The listing builds one solid part. Answer for the finished solid, in the listing's coordinates (mm). A direction names the side the tool comes from. Round coordinates to 2 decimals unless told otherwise and drop trailing zeros. Loops run counter-clockwise (first coordinate to the right, second up) from the corner with the lowest first, then second, coordinate; pieces in that order, holes last. Notation, with made-up numbers: (-4, 41) -> (2, 41) arc R27 cw to (2, 57) -> close; hole circle Ø2 at (-27.5, 69). An arc over 180 degrees is marked (long way). One line per question, with ' | ' between items.
from build123d import *

# Parameters (mm, degrees)
PAD_DEPTH       = 40
SKETCH002_R     = 6.5
PAD001_DEPTH    = 3.25
SKETCH003_R     = 3.5
POCKET_DEPTH    = 8.251
SKETCH004_R     = 3
POCKET001_DEPTH = 5
CHAMFER_SIZE    = 2
FILLET_R        = 2
FILLET001_R     = 2
CHAMFER001_SIZE = 1


with BuildPart() as part:
    # Sketch → Pad (new body)
    with BuildSketch(Plane.XY):
        Polygon((0, 50), (0, 0), (-50, 0), (-50, 5), (-5, 5), (-5, 50), align=None)
    extrude(amount=PAD_DEPTH)

    # Sketch002 (on Face4 of Pad) → Pad001 (join)
    with BuildSketch(Plane(origin=(0, 5, 0), x_dir=(-1, 0, 0), z_dir=(0, 1, 0))):
        with Locations((25, 20)):
            Circle(SKETCH002_R)
    extrude(amount=PAD001_DEPTH)

    # Sketch003 (on Face10 of Pad001) → Pocket (cut, through all)
    with BuildSketch(Plane(origin=(0, 8.25, 0), x_dir=(-1, 0, 0), z_dir=(0, 1, 0))):
        with Locations((25, 20)):
            Circle(SKETCH003_R)
    extrude(amount=-POCKET_DEPTH, mode=Mode.SUBTRACT)

    # Sketch004 (on Face6 of Pocket) → Pocket001 (cut)
    with BuildSketch(Plane(origin=(-5, 0, 0), x_dir=(0, -1, 0), z_dir=(-1, 0, 0))):
        with Locations((-35, 30)):
            Circle(SKETCH004_R)
        with Locations((-20, 10)):
            Circle(SKETCH004_R)
    extrude(amount=-POCKET001_DEPTH, mode=Mode.SUBTRACT)

    # Chamfer
    chamfer_edges = [part.edges().sort_by_distance(p)[0] for p in [
        (-5, 23, 10),
        (-5, 38, 30),
    ]]
    chamfer(chamfer_edges, length=CHAMFER_SIZE)

    # Fillet
    fillet_edges = [part.edges().sort_by_distance(p)[0] for p in [
        (-50, 2.5, 40),
        (-50, 2.5, 0),
    ]]
    fillet(fillet_edges, radius=FILLET_R)

    # Fillet001
    fillet001_edges = [part.edges().sort_by_distance(p)[0] for p in [
        (-2.5, 50, 40),
        (-2.5, 50, 0),
    ]]
    fillet(fillet001_edges, radius=FILLET001_R)

    # Chamfer001
    chamfer001_edges = [part.edges().sort_by_distance(p)[0] for p in [
        (-18.5, 8.25, 20),
    ]]
    chamfer(chamfer001_edges, length=CHAMFER001_SIZE)


solid = part.part
Q1. For faces 1 (the face through (-2, 38, 30)), 2 (the face through (-25, 8.25, 16)), 3 (the face through (-20.209, 6.109, 24.393)), determine the directions among +Z, -Z, +X, -X, +Y, -Y from which every point of the face is accessible in a straight line to the end or side of a thin tool.
Numbers:
face 1: +X, -X | face 2: +Z, -Z, -X, +Y | face 3: +Y
Q2. Find the intervals of material crossed by line 1 (Z direction, x = -25, y = 6); line 2 (Z direction, x = -1, y = 20); line 3 (X direction, y = 12, z = 19), in increasing order. Write a range as from..to.
Numbers:
line 1: 13.5..16.5, 23.5..26.5 | line 2: 0..7, 13..40 | line 3: -5..0
Q3. A cutting plane is placed at D-D on y = 35. Give the vertices of the cut face in (x, z), plus the area to 3 significant figures.
Numbers:
outline: (-5, 0) -> (0, 0) -> (0, 27) -> (-3, 27) -> (-5, 25) -> close; (-5, 35) -> (-3, 33) -> (0, 33) -> (0, 40) -> (-5, 40) -> close | area: 166 mm^2
Q4. A cutting plane is placed at B-B on y = 6.5. Give the vertices of the cut face in (x, z), plus the area to 3 significant figures.
Numbers:
outline: circle Ø13 at (-25, 20); (-5, 0) -> (0, 0) -> (0, 40) -> (-5, 40) -> close; hole circle Ø7 at (-25, 20) | area: 294 mm^2
Q5. For a pull along Z with two mould halves and no side action, classify faces 4 (the face through (-2, 23, 10)), 5 (the face through (-2.46, 49.4, 0.57)), 6 (the face through (-3.125, 20.677, 6.949)), 7 (the face through (-2.46, 49.43, 39.4)) as pulls with the +Z half, pulls with the -Z half, needs draft (parallel to the pull), parting line crosses it, or undercut.
Numbers:
face 4: undercut | face 5: pulls with the -Z half | face 6: undercut | face 7: pulls with the +Z half
Q6. A cutting plane is placed at A-A on x = -25. Give the vertices of the cut face in (y, z), plus the area to 4 significant figures.
Numbers:
outline: (0, 0) -> (5, 0) -> (5, 13.5) -> (7.25, 13.5) -> (8.25, 14.5) -> (8.25, 16.5) -> (0, 16.5) -> close; (0, 23.5) -> (8.25, 23.5) -> (8.25, 25.5) -> (7.25, 26.5) -> (5, 26.5) -> (5, 40) -> (0, 40) -> close | area: 183.5 mm^2
Q7. A cutting plane is placed at C-C on z = 20. Give the vertices of the cut face in (x, y), plus the area to 4 significant figures.
Numbers:
outline: (-50, 0) -> (-28.5, 0) -> (-28.5, 8.25) -> (-30.5, 8.25) -> (-31.5, 7.25) -> (-31.5, 5) -> (-50, 5) -> close; (-21.5, 0) -> (0, 0) -> (0, 50) -> (-5, 50) -> (-5, 5) -> (-18.5, 5) -> (-18.5, 7.25) -> (-19.5, 8.25) -> (-21.5, 8.25) -> close | area: 458.5 mm^2
Q8. Given pin 1 Ø6 at (y, z) = (21.5, 14.5) entering from -X; pin 2 Ø3 at (x, z) = (-15, 35) entering from +Y; pin 3 Ø9 at (x, z) = (-25, 20) entering from +Y, each flat-ended and moving along its own axis, determine where each tip first touches the part or whether it passes through.
Numbers:
pin 1: x = -5 | pin 2: y = 5 | pin 3: y = 8.25
